The model under review builds one solid part; all positions refer to its coordinate system, in mm. Face numbers are marked on the shaded views. A direction names the side the tool comes from. Round coordinates to 2 decimals unless told otherwise and drop trailing zeros. Order: outer loops, then holes, each group sorted by start corner. A loop starts at its lowest first (then second) coordinate and runs counter-clockwise, first axis right, second up. Notation, with made-up numbers: M 9,35.25 L 58,35.25 A8 cw 58,40.25 Z; hole C 89.25,5.5 d7. An arc over 180 degrees is marked long. Answer as a JSON object with one key per item and string values. Group by question number.
1) Insertion check: pin 1 Ø1.5 at (x, z) = (-1.5, -23) entering from +Y; pin 2 Ø0.9 at (x, z) = (1, 4) entering from -Y; pin 3 Ø3 at (y, z) = (2.5, -5) entering from +X. Each pin has a flat end and moves straight along its axis. Give the tip position at first contact, or say it passes through.
2) To check wall thickness, follow line 1 (Z direction, x = -3.5, y = 1.5); line 2 (Z direction, x = 4, y = -1.25); line 3 (Y direction, x = -0.25, z = -19). State the ranges of each line that lie inside material, in increasing order.
3) For the marked faces 1, 2 and 3, list the 3-axis set-ups (+Z, -Z, +X, -X, +Y, -Y) from which the entire face can be reached by the end or side of a thin tool; tool diameter is ignored.
4) Consider section A-A, the plane x = 0. Write out the cut boundary in (y, z), then the cut area to 3 significant figures.
5) Consider section B-B, the plane z = -2. Write out the cut boundary in (x, y).
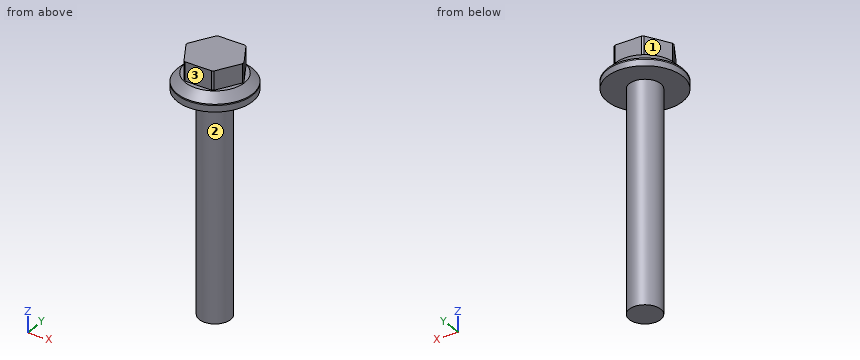
```python
from build123d import *

# Parameters (mm, degrees)
SKETCH1_W                = 2.5
SKETCH1_H                = 35
SKETCH2_R                = 6
BOSS_EXTRUDE1_DEPTH      = 1
SKETCH3_R                = 4.4
BOSS_EXTRUDE2_DEPTH      = 1.5
CHAMFER1_SIZE            = 1.8
BOSS_EXTRUDE3_DEPTH      = 3
BOSS_EXTRUDE3_DEPTH_BACK = 1.5
CHAMFER2_SIZE            = 0.2
CHAMFER2_EDGE_2_SIZE     = 0.2
CHAMFER2_EDGE_3_SIZE     = 0.2
CHAMFER2_EDGE_4_SIZE     = 0.2
CHAMFER2_EDGE_5_SIZE     = 0.2
CHAMFER2_EDGE_6_SIZE     = 0.2


with BuildPart() as part:
    # Sketch1 → Revolve1 (revolve)
    with BuildSketch(Plane(origin=(0, 0, 0), x_dir=(1, 0, 0), z_dir=(0, 1, 0)), mode=Mode.PRIVATE) as revolve1_sk:
        with Locations((1.25, 17.5)):
            Rectangle(SKETCH1_W, SKETCH1_H)
    revolve(revolve1_sk.sketch.rotate(Axis((0, 0, -35), (0, 0, 1)), 180), axis=Axis((0, 0, -35), (0, 0, 1)))

    # Sketch2 → Boss-Extrude1 (add)
    with BuildSketch(Plane.XY):
        Circle(SKETCH2_R)
    extrude(amount=BOSS_EXTRUDE1_DEPTH)

    # Sketch3 → Boss-Extrude2 (add)
    with BuildSketch(Plane.XY.offset(1)):
        Circle(SKETCH3_R)
    extrude(amount=BOSS_EXTRUDE2_DEPTH)

    # Chamfer1
    # the kernel refuses this chamfer: 1.8 mm, written as the material it adds along each edge
    with BuildSketch(Plane(origin=(0, 0, 1), x_dir=(1, 0, 0), z_dir=(0, -1, 0))) as chamfer1_piece_1_section:
        Polygon((4.4 + CHAMFER1_SIZE, 0), (4.4, CHAMFER1_SIZE), (4.4, 0), align=None)
    chamfer1_piece_1 = revolve(axis=Axis((0, 0, 1), (0, 0, 1)), mode=Mode.PRIVATE)
    chamfer1_piece_1 = chamfer1_piece_1 & Plane(origin=(0, 0, 1.82351745), x_dir=(1, 0, 0), z_dir=(0, 0, -1)) * Cylinder(6, 25, mode=Mode.PRIVATE)
    chamfer1_piece_1 = split(chamfer1_piece_1, bisect_by=Plane(origin=(-5.32351745, 0, 2.5), z_dir=(0, 0, -1)), keep=Keep.TOP, mode=Mode.PRIVATE)
    add(chamfer1_piece_1)

    # Sketch4 → Boss-Extrude3 (add, two sides: drawn at the far end of the back side and taken through both)
    with BuildSketch(Plane.XY.offset(2.5).offset(-BOSS_EXTRUDE3_DEPTH_BACK)):
        Polygon((-2.309401077, 4), (-4.618802154, 0), (-2.309401077, -4), (2.309401077, -4), (4.618802154, 0), (2.309401077, 4), align=None)
    extrude(amount=BOSS_EXTRUDE3_DEPTH + BOSS_EXTRUDE3_DEPTH_BACK)

    # Chamfer2
    chamfer2_edges = [part.edges().sort_by_distance(p)[0] for p in [
        (-2.309401077, 4, 4),
    ]]
    chamfer(chamfer2_edges, length=CHAMFER2_SIZE)

    # Chamfer2 edge 2
    chamfer2_edge_2_edges = [part.edges().sort_by_distance(p)[0] for p in [
        (2.309401077, 4, 4),
    ]]
    chamfer(chamfer2_edge_2_edges, length=CHAMFER2_EDGE_2_SIZE)

    # Chamfer2 edge 3
    chamfer2_edge_3_edges = [part.edges().sort_by_distance(p)[0] for p in [
        (4.618802154, 0, 4),
    ]]
    chamfer(chamfer2_edge_3_edges, length=CHAMFER2_EDGE_3_SIZE)

    # Chamfer2 edge 4
    chamfer2_edge_4_edges = [part.edges().sort_by_distance(p)[0] for p in [
        (2.309401077, -4, 4),
    ]]
    chamfer(chamfer2_edge_4_edges, length=CHAMFER2_EDGE_4_SIZE)

    # Chamfer2 edge 5
    chamfer2_edge_5_edges = [part.edges().sort_by_distance(p)[0] for p in [
        (-2.309401077, -4, 4),
    ]]
    chamfer(chamfer2_edge_5_edges, length=CHAMFER2_EDGE_5_SIZE)

    # Chamfer2 edge 6
    chamfer2_edge_6_edges = [part.edges().sort_by_distance(p)[0] for p in [
        (-4.618802154, 0, 4),
    ]]
    chamfer(chamfer2_edge_6_edges, length=CHAMFER2_EDGE_6_SIZE)


solid = part.part
```
Results list:
{
 "1": {"pin 1": "y = 2.38", "pin 2": "y = -4", "pin 3": "x = 2.29"},
 "2": {"line 1": "0 to 5.5", "line 2": "0 to 2.5", "line 3": "-2.49 to 2.49"},
 "3": {"face 1": "+Z, -X, +Y", "face 2": "-Z", "face 3": "+Z, +X, -X, -Y"},
 "4": {"outline": "M -6,0 L -2.5,0 L -2.5,-35 L 2.5,-35 L 2.5,0 L 6,0 L 6,1.2 L 4.7,2.5 L 4,2.5 L 4,5.5 L -4,5.5 L -4,2.5 L -4.7,2.5 L -6,1.2 Z", "area": "227 mm^2"},
 "5": {"outline": "C 0,0 d5"}
}
